Autodesk Inventor part; units mm, degrees
ref_plane "YZ Plane" through (0, 0, 0) normal (1, 0, 0) x (0, 1, 0)
ref_plane "XZ Plane" through (0, 0, 0) normal (0, 1, 0) x (-1, 0, 0)
ref_plane "XY Plane" through (0, 0, 0) normal (0, 0, 1) x (1, 0, 0)
sketch "スケッチ1" plane through (0, 0, 0) normal (0, 0, 1) x (1, 0, 0)
  line L0 (0, 0) -> (20, 0)
  line L1 (20, 0) -> (20, 1.5)
  line L2 (20, 1.5) -> (0, 1.5)
  line L3 (0, 1.5) -> (0, 0)
  line L4 (0, 0) -> (0, 2.75)
  line L5 (0, 0) -> (-2, 0)
  line L6 (-2, 0) -> (0, 0)
  line L7 (-2, 0) -> (-2, 1.15)
  arc A0 (0, 2.75) -> (-2, 1.15) centre (-0.0403, 0.7504) ccw
  dimension "d0" = 1.5
  dimension "d1" = 20
  dimension "d3" = 2
  dimension "d4" = 2.75
  dimension "d5" = 1.15
  dimension "d6" = 2
revolve "回転1" add sketch "スケッチ1" angle 360 about axis through (-2, 0, 0) along (1, 0, 0)
thread "ねじ1"
sketch "スケッチ2" plane through (-2, 0, 0) normal (-1, 0, 0) x (0, 0, 1)
  circle A0 centre (0, 0) radius 1.15
  line L0 (-0.575, 0.9959) -> (0.575, 0.9959)
  line L1 (0.575, 0.9959) -> (1.15, 0)
  line L2 (1.15, 0) -> (0.575, -0.9959)
  line L3 (0.575, -0.9959) -> (-0.575, -0.9959)
  line L4 (-0.575, -0.9959) -> (-1.15, 0)
  line L5 (-1.15, 0) -> (-0.575, 0.9959)
  dimension "d10" = 1.15
  dimension "d11" = 1.9919
extrude "押し出し1" cut sketch "スケッチ2" against normal blind 1.4 contours L2 L3 L4 L5 L0 L1
fillet "フィレット1" radius 0.2 6 edges at (-0.6, 0.9959, 0) (-0.6, 0.498, 0.8625) (-0.6, 0.498, -0.8625) (-0.6, -0.498, -0.8625) (-0.6, -0.9959, 0) (-0.6, -0.498, 0.8625)
fillet "フィレット2" radius 0.1 1 edges at (0, -1.5, 0)
fillet "フィレット3" radius 0.1 1 edges at (20, -1.5, 0)
properties part number "ネジボタンM3L20" material "鋼"
Verification items for the finished model (mm, model axes). A direction names the side the tool comes from. Round coordinates to 2 decimals unless told otherwise and drop trailing zeros. Loops run counter-clockwise (first coordinate to the right, second up) from the corner with the lowest first, then second, coordinate; pieces in that order, holes last. Notation, with made-up numbers: (42, -15.5) - (101, -15.5) arc R17 ccw to (101, -8.5) - close; hole circle Ø11 at (14.25, -14). An arc over 180 degrees is marked (long way). Use a Markdown table: item, result. Add a question column.
1. Section check A-A, the plane x = 11.5. Record the boundary of the cut face in (y, z).
2. Release check for a two-part mould opening along Y. For faces 1 (the face through (-1, 0.996, 0)), 2 (the face through (0, 2, 0)), 3 (the face through (9.86, -1.5, -0.07)) record: released by +Y, released by -Y, zero draft, split by the parting line, or undercut.
3. Thickness scan on probe 1 along Z at (x, y) = (12.75, 0.1); probe 2 along X at (y, z) = (-0.75, 0.9); probe 3 along Y at (x, z) = (-0.75, 0.95). Record the ranges inside material, lowest first. Write a range as [from, to].
4. Gauge pin test, flat ends, axial feed: pin 1 (1.3 mm diameter, centred on x = -1.5, z = 0, fed in from -Y); pin 2 (0.6 mm diameter, centred on x = -1, z = 0, fed in from +Y); pin 3 (1.3 mm diameter, centred on y = 0, z = 0, fed in from -X). Record the tip position at first contact, or that the pin passes through.
5. Access from +Z, -Z, +X, -X, +Y, -Y to the whole of each face (thin tool, end or side, straight path). Record for faces 4 (the face through (-1.408, 0.491, -0.867)), 5 (the face through (20, 0, 0)).
Checks:
| question | item | result |
|---|---|---|
| 1 | outline | circle Ø3 at (0, 0) |
| 2 | face 1 | undercut |
| 2 | face 2 | zero draft |
| 2 | face 3 | split by the parting line |
| 3 | probe 1 | z = [-1.5, 1.5] |
| 3 | probe 2 | x = [-2, 20] |
| 3 | probe 3 | y = [-2.44, -0.33], [0.33, 2.44] |
| 4 | pin 1 | stops at y = -2.58 |
| 4 | pin 2 | stops at y = 2.64 |
| 4 | pin 3 | stops at x = -0.6 |
| 5 | face 4 | -X |
| 5 | face 5 | +Z, -Z, +X, +Y, -Y |
